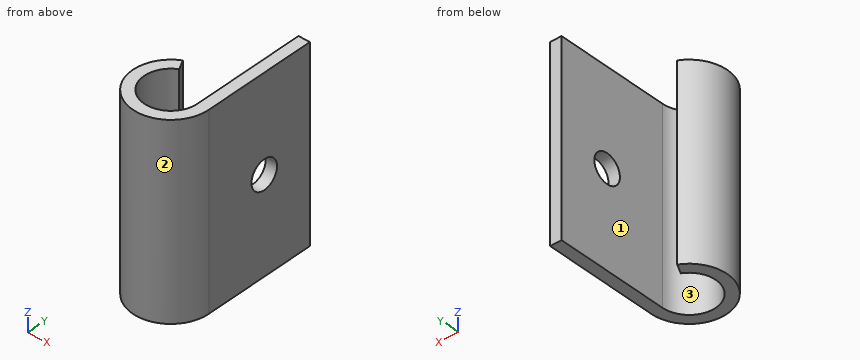
```python
from build123d import *

# Parameters (mm, degrees)
F1_DEPTH = 25
F3_D     = 3.8
F3_DEPTH = 20


with BuildPart() as f1:
    # F0 (on Top) → F1 (new body)
    with BuildSketch(Plane.XY):
        with BuildLine():
            ThreePointArc((3.5, 0), (-1.804479, -2.998976), (-1.639346, 3.092337))
            Line((-1.639346, 3.092337), (-2.341922, 4.417624))
            ThreePointArc((-2.341922, 4.417624), (-2.577827, -4.284251), (5, 0))
            Line((5, 0), (5, 15))
            Line((5, 15), (3.5, 15))
            Line((3.5, 15), (3.5, 0))
        make_face()
    extrude(amount=F1_DEPTH)

    # F3
    with Locations(Plane(origin=(3.5, 0, 0), x_dir=(0, -1, 0), z_dir=(-1, 0, 0))):
        with Locations((-8.230869, 12.5)):
            Hole(F3_D / 2, depth=F3_DEPTH)


solid = f1.part
```
Source: CAD feature listing. Evaluate the final solid. Frame: model axes, mm. Face numbers are marked on the shaded views. Give positions to 0.01 mm unless a question says otherwise; leave off trailing zeros. Loops run counter-clockwise (first coordinate to the right, second up) from the corner with the lowest first, then second, coordinate; pieces in that order, holes last. Notation, with made-up numbers: (89, 44) -> (108, 44) arc R21 ccw to (108, 52) -> close; hole circle Ø1 at (-25, 10.5). An arc over 180 degrees is marked (long way). Use a Markdown table: item, result. Add a question column.
(1) Ray query, line 1 (X direction, y = 7.25, z = 9.25); line 2 (X direction, y = 2.25, z = 19.5); line 3 (Y direction, x = -2.25, z = 8.75). Return the intervals inside material, ascending.
(2) Section query C-C (x = -3). Output: boundary loops of the cut face in (y, z).
(3) First-contact query: pin 1 Ø8 at (y, z) = (0.5, 15.5) entering from -X; pin 2 Ø2 at (x, z) = (1.5, 10.5) entering from -Y; pin 3 Ø2 at (y, z) = (4.5, 4.5) entering from -X. Flat tips, straight axial feed; report the tip coordinate or a pass-through.
(4) Section query B-B (y = 0.5). Output: boundary loops of the cut face in (x, z), then the cut area to 3 significant figures.
(5) Section query A-A (z = 12.5). Output: boundary loops of the cut face in (x, y).
(6) Pull-direction query (Y, two-part tool) for the marked faces 1, 2 and 3; classes: +Y half, -Y half, draft (parallel to the pull), parting line (faces both ways), or undercut.
(7) Section query D-D (z = 17.5). Output: boundary loops of the cut face in (x, y).
Checked values:
| question | item | result |
|---|---|---|
| 1 | line 1 | 3.5 to 5 |
| 1 | line 2 | -4.47 to -2.68, 3.5 to 5 |
| 1 | line 3 | -4.47 to -2.68, 2.68 to 4.24 |
| 2 | outline | (-4, 0) -> (-1.8, 0) -> (-1.8, 25) -> (-4, 25) -> close; (1.8, 0) -> (4, 0) -> (4, 25) -> (1.8, 25) -> close |
| 3 | pin 1 | x = -5 |
| 3 | pin 2 | y = -4.97 |
| 3 | pin 3 | x = -3.57 |
| 4 | outline | (-4.97, 0) -> (-3.46, 0) -> (-3.46, 25) -> (-4.97, 25) -> close; (3.5, 0) -> (5, 0) -> (5, 25) -> (3.5, 25) -> close |
| 4 | area | 75.3 mm^2 |
| 5 | outline | (-2.34, 4.42) arc R5 ccw (long way) to (5, 0) -> (5, 6.33) -> (3.5, 6.33) -> (3.5, 0) arc R3.5 cw (long way) to (-1.64, 3.09) -> close; (3.5, 10.13) -> (5, 10.13) -> (5, 15) -> (3.5, 15) -> close |
| 6 | face 1 | draft |
| 6 | face 2 | parting line |
| 6 | face 3 | undercut |
| 7 | outline | (-2.34, 4.42) arc R5 ccw (long way) to (5, 0) -> (5, 15) -> (3.5, 15) -> (3.5, 0) arc R3.5 cw (long way) to (-1.64, 3.09) -> close |
